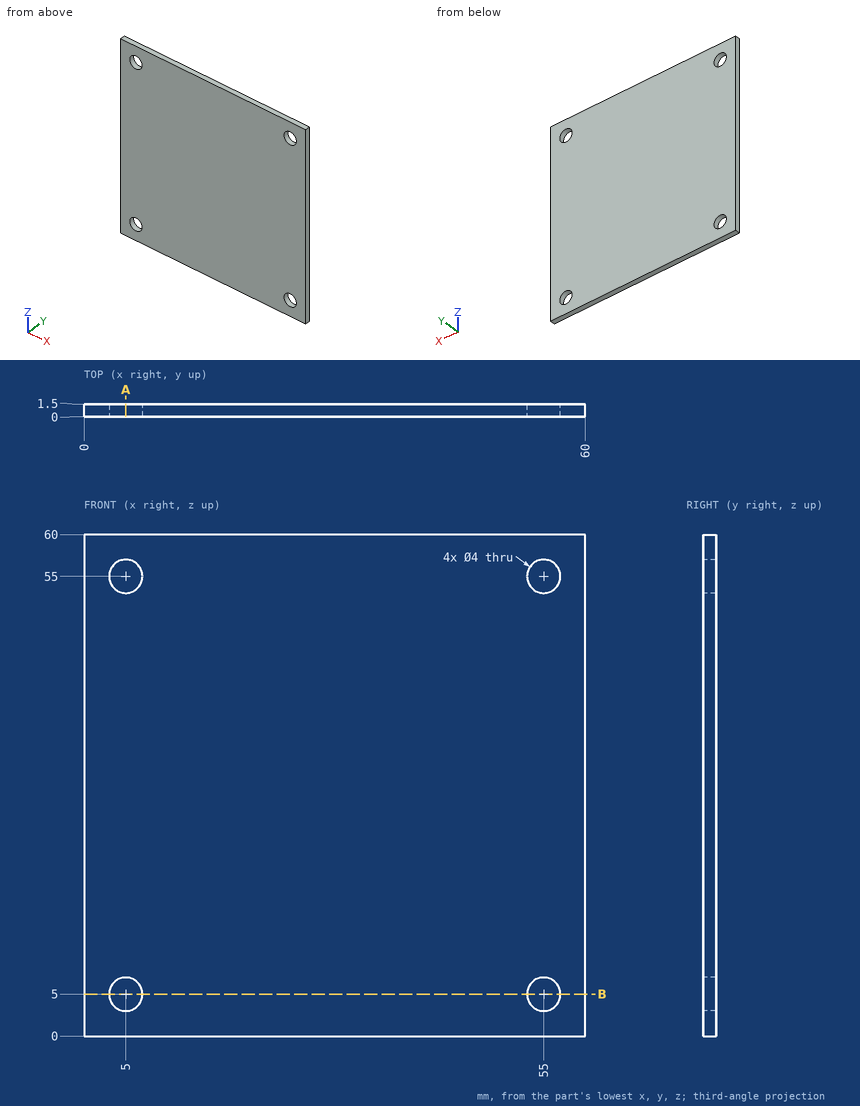
Could you check a few things on this drawing? It's one solid part, dimensions in mm from its lowest x, y, z. Coordinates: 2 decimals unless noted, no trailing zeros. Order: outer loops, then holes, each group sorted by start corner. A loop starts at its lowest first (then second) coordinate and runs counter-clockwise, first axis right, second up. Notation, with made-up numbers: M -12,3 L 32,3 A18 ccw 32,33 Z; hole C 30,-4.5 d9. An arc over 180 degrees is marked long. Use a Markdown table: item, result. Add a question column.
Q1. I'm going to push a flat-ended pin straight in: pin 1 (3 mm diameter, centred on x = 5, z = 5, fed in from +Y). Where does the tip first touch, or does it pass through?
Q2. I want a section at B-B on z = 5. List the corners of the cut face in (x, y) for me, then the cut area to 3 significant figures.
Q3. If I drill on L1, parallel to Z at x = 5, y = 0.6; L2, parallel to Z at x = 54, y = 1, over which ranges is the centre line in solid material (lowest first)?
Q4. I want a section at A-A on x = 5. List the corners of the cut face in (y, z) for me, then the cut area to 3 significant figures.
Checked values:
| question | item | result |
|---|---|---|
| 1 | pin 1 | through |
| 2 | outline | M 0,0 L 3,0 L 3,1.5 L 0,1.5 Z; M 7,0 L 53,0 L 53,1.5 L 7,1.5 Z; M 57,0 L 60,0 L 60,1.5 L 57,1.5 Z |
| 2 | area | 78.0 mm² |
| 3 | L1 | 0 to 3, 7 to 53, 57 to 60 |
| 3 | L2 | 0 to 3.27, 6.73 to 53.27, 56.73 to 60 |
| 4 | outline | M 0,0 L 1.5,0 L 1.5,3 L 0,3 Z; M 0,7 L 1.5,7 L 1.5,53 L 0,53 Z; M 0,57 L 1.5,57 L 1.5,60 L 0,60 Z |
| 4 | area | 78.0 mm² |
